The drawing under review shows one solid part. Ordinate dimensions are in mm from its lowest x, y, z. A direction names the side the tool comes from. Coordinates: 2 decimals unless noted, no trailing zeros. Write each loop counter-clockwise with the first axis right and the second up, starting at its lowest first coordinate (ties: lowest second). Pieces come first, ordered by that corner, then holes.
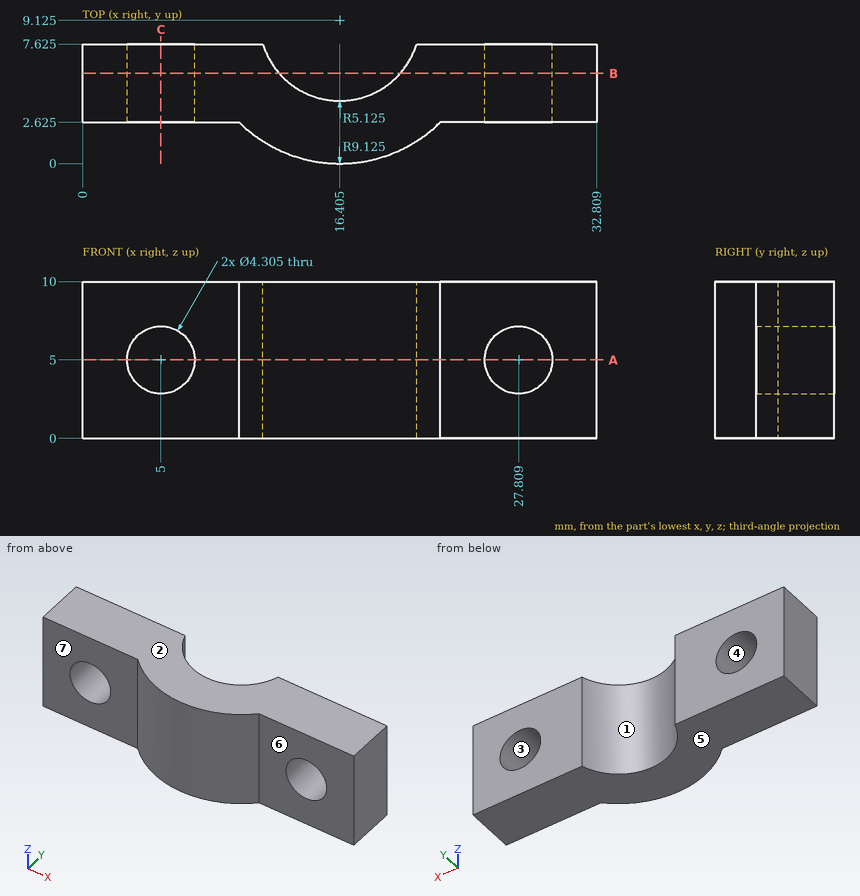
Q1. Tool access review of the marked faces 5, 6 and 7: name each direction out of +Z, -Z, +X, -X, +Y, -Y from which nothing blocks a thin tool from reaching the whole face with its end or side.
Ans:
face 5: -Z, +X, -X, +Y, -Y
face 6: +Z, -Z, +X, -Y
face 7: +Z, -Z, -X, -Y
Q2. Draft analysis for pull direction Z (two halves, no side actions). For the marked faces 1, 2, 3 and 4, state which applies: +Z half, -Z half, draft (parallel to the pull), parting line (faces both ways), or undercut.
Ans:
face 1: draft
face 2: +Z half
face 3: undercut
face 4: undercut
Q3. For probe 1 along Z at (x, y) = (5, 6.45); probe 2 along X at (y, z) = (5.5, 4) (1 decimal); probe 3 along X at (y, z) = (2.75, 4.5) (1 decimal), list the stretches that pass through material, from the lowest coordinate up.
Ans:
probe 1: z = 0 to 2.85, 7.15 to 10
probe 2: x = 0 to 3.1, 6.9 to 12.8, 20 to 25.9, 29.7 to 32.8
probe 3: x = 0 to 2.9, 7.1 to 25.7, 29.9 to 32.8
Q4. Add section C-C (x = 5). State the section outline as (y, z) points (1 decimal).
Ans:
outline: (2.6, 0) - (7.6, 0) - (7.6, 2.8) - (2.6, 2.8) - close; (2.6, 7.2) - (7.6, 7.2) - (7.6, 10) - (2.6, 10) - close
Q5. Add section B-B (y = 5.75). State the section outline as (x, z) points (1 decimal).
Ans:
outline: (0, 0) - (12.5, 0) - (12.5, 10) - (0, 10) - close; (20.3, 0) - (32.8, 0) - (32.8, 10) - (20.3, 10) - close; hole circle Ø4.3 at (5, 5); hole circle Ø4.3 at (27.8, 5)
Q6. Add section A-A (z = 5). Give the number of separate pieces and of enclosed holes in the cut face, then the cut area to 3 significant figures.
Ans:
separate pieces: 3
enclosed holes: 0
area: 118 mm2
Q7. Clearance check with flat-ended pins moving along their axes: pin 1 Ø5 at (x, z) = (29.5, 3.5) entering from -Y (1 decimal); pin 2 Ø4 at (x, z) = (14.5, 4) entering from +Y (1 decimal); pin 3 Ø3.5 at (x, z) = (5, 5) entering from +Y; pin 4 Ø6 at (x, z) = (3.5, 5) entering from +Y (1 decimal). State where each tip first meets the part, or that it passes through.
Ans:
pin 1: stops at y = 2.6
pin 2: stops at y = 5.8
pin 3: passes through
pin 4: stops at y = 7.6
